Here's how the part is built. I have some questions about the finished solid (model axes, mm). Coordinates: 2 decimals unless noted, no trailing zeros. Write each loop counter-clockwise with the first axis right and the second up, starting at its lowest first coordinate (ties: lowest second). Pieces come first, ordered by that corner, then holes.
```python
from build123d import *

# Parameters (mm, degrees)
SKETCH1_W                                    = 75
SKETCH1_H                                    = 47
BOSS_EXTRUDE1_DEPTH                          = 2
SKETCH3_R                                    = 4
CUT_EXTRUDE1_DEPTH                           = 5
CSK_FOR_M2_COUNTERSUNK_FLAT_HEAD_SCR_2_COUNT = 2
CSK_FOR_M2_COUNTERSUNK_FLAT_HEAD_SCR_2_PITCH = 24.5
CSK_FOR_M2_COUNTERSUNK_FLAT_HEAD_SCR_3_COUNT = 2
CSK_FOR_M2_COUNTERSUNK_FLAT_HEAD_SCR_3_PITCH = 65
CSK_FOR_M2_COUNTERSUNK_FLAT_HEAD_SCR_4_COUNT = 2
CSK_FOR_M2_COUNTERSUNK_FLAT_HEAD_SCR_4_PITCH = 69.464019463


with BuildPart() as part:
    # Sketch1 → Boss-Extrude1 (new body)
    with BuildSketch(Plane.XY):
        Rectangle(SKETCH1_W, SKETCH1_H)
    extrude(amount=BOSS_EXTRUDE1_DEPTH)

    # Sketch3 → Cut-Extrude1 (cut)
    with BuildSketch(Plane.XY.offset(2)):
        with Locations((0, -4)):
            Circle(SKETCH3_R)
    extrude(amount=-CUT_EXTRUDE1_DEPTH, mode=Mode.SUBTRACT)

    # Sketch5 → CSK for M2 Countersunk Flat Head Screw1 (revolve, cut)
    with BuildSketch(Plane(origin=(32.5, 8.5, 0), x_dir=(0, 1, 0), z_dir=(1, 0, 0))):
        Polygon((0, 0), (0, 2), (1.2, 2), (1.2, 1), (2.2, 0), align=None)
    csk_for_m2_countersunk_flat_head_screw1 = revolve(axis=Axis((32.5, 8.5, -6.35), (0, 0, 1)), mode=Mode.SUBTRACT)

    # CSK for M2 Countersunk Flat Head Scr 2: CSK for M2 Countersunk Flat Head Screw1 ×2
    with Locations(*[(0, -i * CSK_FOR_M2_COUNTERSUNK_FLAT_HEAD_SCR_2_PITCH, 0) for i in range(1, CSK_FOR_M2_COUNTERSUNK_FLAT_HEAD_SCR_2_COUNT)]):
        add(csk_for_m2_countersunk_flat_head_screw1, mode=Mode.SUBTRACT)

    # CSK for M2 Countersunk Flat Head Scr 3: CSK for M2 Countersunk Flat Head Screw1 ×2
    with Locations(*[(-i * CSK_FOR_M2_COUNTERSUNK_FLAT_HEAD_SCR_3_PITCH, 0, 0) for i in range(1, CSK_FOR_M2_COUNTERSUNK_FLAT_HEAD_SCR_3_COUNT)]):
        add(csk_for_m2_countersunk_flat_head_screw1, mode=Mode.SUBTRACT)

    # CSK for M2 Countersunk Flat Head Scr 4: CSK for M2 Countersunk Flat Head Screw1 ×2
    with Locations(*[Vector(-0.935736234, -0.352700581, 0) * (i * CSK_FOR_M2_COUNTERSUNK_FLAT_HEAD_SCR_4_PITCH) for i in range(1, CSK_FOR_M2_COUNTERSUNK_FLAT_HEAD_SCR_4_COUNT)]):
        add(csk_for_m2_countersunk_flat_head_screw1, mode=Mode.SUBTRACT)


solid = part.part
```
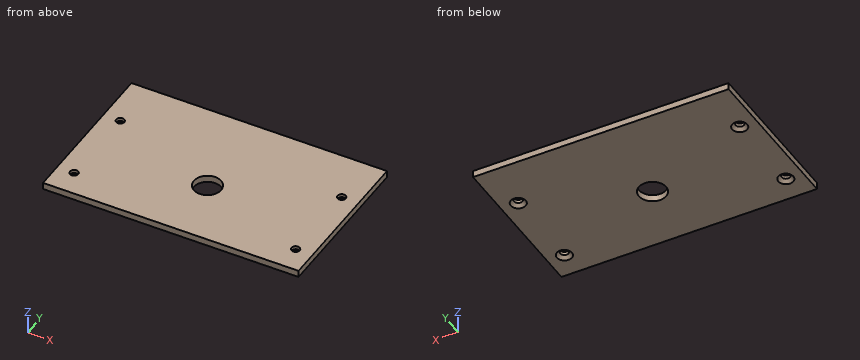
1) Imagine slicing it at D-D on x = 0. Please give me the cut outline in (y, z), then the cut area to 3 significant figures.
Values follow:
outline: (-23.5, 0) - (-8, 0) - (-8, 2) - (-23.5, 2) - close; (0, 0) - (23.5, 0) - (23.5, 2) - (0, 2) - close
area: 78.0 mm2
2) Imagine slicing it at A-A on x = -32.5. Please give me the cut outline in (y, z).
Values follow:
outline: (-23.5, 0) - (-18.2, 0) - (-17.2, 1) - (-17.2, 2) - (-23.5, 2) - close; (-14.8, 1) - (-13.8, 0) - (6.3, 0) - (7.3, 1) - (7.3, 2) - (-14.8, 2) - close; (9.7, 1) - (10.7, 0) - (23.5, 0) - (23.5, 2) - (9.7, 2) - close
3) Imagine slicing it at C-C on y = -16. Please give me the cut outline in (x, z).
Values follow:
outline: (-37.5, 0) - (-34.7, 0) - (-33.7, 1) - (-33.7, 2) - (-37.5, 2) - close; (-31.3, 1) - (-30.3, 0) - (30.3, 0) - (31.3, 1) - (31.3, 2) - (-31.3, 2) - close; (33.7, 1) - (34.7, 0) - (37.5, 0) - (37.5, 2) - (33.7, 2) - close
4) Imagine slicing it at B-B on z = 1.4. Please give me the cut outline in (x, y), then the cut area to 3 significant figures.
Values follow:
outline: (-37.5, -23.5) - (37.5, -23.5) - (37.5, 23.5) - (-37.5, 23.5) - close; hole circle Ø2.4 at (-32.5, -16); hole circle Ø2.4 at (-32.5, 8.5); hole circle Ø8 at (0, -4); hole circle Ø2.4 at (32.5, -16); hole circle Ø2.4 at (32.5, 8.5)
area: 3,460 mm2
5) I need wall thicknesses on probe 1 along X at (y, z) = (8.5, 1.75); probe 2 along Y at (x, z) = (0, 0.4); probe 3 along X at (y, z) = (-6, 1.8). Which ranges of each line are inside material? Lowest first, please.
Values follow:
probe 1: x = -37.5 to -33.7, -31.3 to 31.3, 33.7 to 37.5
probe 2: y = -23.5 to -8, 0 to 23.5
probe 3: x = -37.5 to -3.46, 3.46 to 37.5
6) Will this pin go through, and if not, where does the flat tip stop? pin 1 (4 mm diameter, centred on x = -32.5, y = 8.5, fed in from -Z).
Values follow:
pin 1: stops at z = 0.2
